Check sheet for the modelled part. Datum: model origin and axes. Units: mm. Give positions to 0.01 mm unless a question says otherwise; leave off trailing zeros. Loops run counter-clockwise (first coordinate to the right, second up) from the corner with the lowest first, then second, coordinate; pieces in that order, holes last. Notation, with made-up numbers: (-23, 82) - (29, 82) arc R14 cw to (29, 96) - close; hole circle Ø7 at (82.25, 19). An arc over 180 degrees is marked (long way). Answer in a Markdown table with one row per item. Add a question column.
(1) Go/stop test with a flat-tipped pin: P1, Ø1, axis at x = -98.5, z = 2, coming from the +Y side. Record where the tip stops, or that it passes through.
(2) Sectioned sample at C-C on z = 0.85. State how many separate pieces and enclosed holes the cut face has, then the cut area to 3 significant figures.
(3) Sectioned sample at B-B on x = -0.5. Enter the section's corners in (y, z).
(4) Thickness scan on L1, parallel to Y at x = -44.5, z = 0.6; L2, parallel to Y at x = 35, z = 1.3; L3, parallel to Y at x = -6.5, z = 2.15. Record the ranges inside material, lowest first.
(5) Sectioned sample at A-A on x = -146.5. Enter the section's corners in (y, z), then the cut area to 3 significant figures.
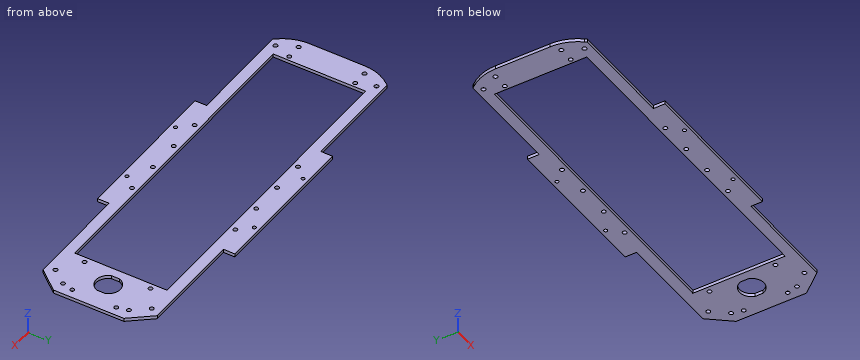
from build123d import *

# Parameters (mm, degrees)
BOSS_EXTRUDE1_DEPTH            = 3
SKETCH2_W                      = 285
SKETCH2_H                      = 84
CUT_EXTRUDE1_DEPTH             = 3
SKETCH3_R                      = 1.95
SKETCH3_R_2                    = 1.6
CUT_EXTRUDE2_DEPTH             = 3
CUT_EXTRUDE3_DEPTH             = 3
SKETCH5_R                      = 1.9
CUT_EXTRUDE4_DEPTH             = 3
SKETCH7_W                      = 36.585559037
SKETCH7_H                      = 111.194930045
CUT_EXTRUDE5_DEPTH             = 10
FILLET1_R                      = 40
SKETCH6_R                      = 1.9
EXPANSION_MOUNTING_HOLES_DEPTH = 10


with BuildPart() as part:
    # Sketch1 → Boss-Extrude1 (new body)
    with BuildSketch(Plane.XY):
        Polygon((-70, 89.297239119), (70, 89.297239119), (70, 78.797239119), (165, 78.797239119), (181.5, 58.797239119), (181.5, -5.202760881), (165, -25.202760881), (70, -25.202760881), (70, -35.702760881), (-70, -35.702760881), (-70, -25.202760881), (-165, -25.202760881), (-181.5, -5.202760881), (-181.5, 58.797239119), (-165, 78.797239119), (-70, 78.797239119), align=None)
    extrude(amount=BOSS_EXTRUDE1_DEPTH)

    # Sketch2 → Cut-Extrude1 (cut)
    with BuildSketch(Plane.XY.offset(3)):
        with Locations((-7.5, 26.797239119)):
            Rectangle(SKETCH2_W, SKETCH2_H)
    extrude(amount=-CUT_EXTRUDE1_DEPTH, mode=Mode.SUBTRACT)

    # Sketch3 → Cut-Extrude2 (cut)
    with BuildSketch(Plane.XY.offset(3)):
        with Locations((-167.5, -3.202760881)):
            Circle(SKETCH3_R)
        with Locations((-167.5, 56.797239119)):
            Circle(SKETCH3_R)
        with Locations((-35, -31.202760881)):
            Circle(SKETCH3_R_2)
        with Locations((35, -31.202760881)):
            Circle(SKETCH3_R_2)
        with Locations((-35, 84.797239119)):
            Circle(SKETCH3_R_2)
        with Locations((35, 84.797239119)):
            Circle(SKETCH3_R_2)
        with Locations((-159.5, 72.797239119)):
            Circle(SKETCH3_R)
        with Locations((-159.5, -19.202760881)):
            Circle(SKETCH3_R)
    extrude(amount=-CUT_EXTRUDE2_DEPTH, mode=Mode.SUBTRACT)

    # Sketch4 → Cut-Extrude3 (cut)
    with BuildSketch(Plane.XY.offset(3)):
        with BuildLine():
            Line((163.8, 30.531204839), (163.8, 23.063273399))
            ThreePointArc((163.8, 23.063273399), (153.4, 15.747239119), (143, 23.063273399))
            Line((143, 23.063273399), (143, 30.531204839))
            ThreePointArc((143, 30.531204839), (153.4, 37.847239119), (163.8, 30.531204839))
        make_face()
    extrude(amount=-CUT_EXTRUDE3_DEPTH, mode=Mode.SUBTRACT)

    # Sketch5 → Cut-Extrude4 (cut)
    with BuildSketch(Plane.XY.offset(3)):
        with Locations((173.5, 6.797239119)):
            Circle(SKETCH5_R)
        with Locations((173.5, 46.797239119)):
            Circle(SKETCH5_R)
        with Locations((140, 56.797239119)):
            Circle(SKETCH5_R)
        with Locations((140, -3.202760881)):
            Circle(SKETCH5_R)
        with Locations((160, 70.547239119)):
            Circle(SKETCH5_R)
        with Locations((160, -16.952760881)):
            Circle(SKETCH5_R)
    extrude(amount=-CUT_EXTRUDE4_DEPTH, mode=Mode.SUBTRACT)

    # Sketch7 → Cut-Extrude5 (cut)
    with BuildSketch(Plane.XY.offset(3)):
        with Locations((-193.792779519, 34.073054392)):
            Rectangle(SKETCH7_W, SKETCH7_H)
    extrude(amount=-CUT_EXTRUDE5_DEPTH, mode=Mode.SUBTRACT)

    # Fillet1
    fillet1_edges = [part.edges().sort_by_distance(p)[0] for p in [
        (-175.5, 66.069966392, 1.5),
        (-175.5, -12.475488154, 1.5),
    ]]
    fillet(fillet1_edges, radius=FILLET1_R)

    # Sketch6 → Expansion mounting holes (cut)
    with BuildSketch(Plane.XY.offset(3)):
        with Locations((171, 56.797239119)):
            Circle(SKETCH6_R)
        with Locations((171, -3.202760881)):
            Circle(SKETCH6_R)
        with Locations((-154, 56.797239119)):
            Circle(SKETCH6_R)
        with Locations((-154, -3.202760881)):
            Circle(SKETCH6_R)
        with Locations((-45, 73.797239119)):
            Circle(SKETCH6_R)
        with Locations((-45, -20.202760881)):
            Circle(SKETCH6_R)
        with Locations((-15, -20.202760881)):
            Circle(SKETCH6_R)
        with Locations((-15, 73.797239119)):
            Circle(SKETCH6_R)
        with Locations((15, -20.202760881)):
            Circle(SKETCH6_R)
        with Locations((15, 73.797239119)):
            Circle(SKETCH6_R)
        with Locations((45, -20.202760881)):
            Circle(SKETCH6_R)
        with Locations((45, 73.797239119)):
            Circle(SKETCH6_R)
    extrude(amount=-EXPANSION_MOUNTING_HOLES_DEPTH, mode=Mode.SUBTRACT)


solid = part.part
Reply:
| question | item | result |
|---|---|---|
| 1 | P1 | y = 78.8 |
| 2 | separate pieces | 1 |
| 2 | enclosed holes | 28 |
| 2 | area | 15,000 mm^2 |
| 3 | outline | (-35.7, 0) - (-15.2, 0) - (-15.2, 3) - (-35.7, 3) - close; (68.8, 0) - (89.3, 0) - (89.3, 3) - (68.8, 3) - close |
| 4 | L1 | -35.7 to -22.04, -18.37 to -15.2, 68.8 to 71.96, 75.63 to 89.3 |
| 4 | L2 | -35.7 to -32.8, -29.6 to -15.2, 68.8 to 83.2, 86.4 to 89.3 |
| 4 | L3 | -35.7 to -15.2, 68.8 to 89.3 |
| 5 | outline | (-25.2, 0) - (-15.2, 0) - (-15.2, 3) - (-25.2, 3) - close; (68.8, 0) - (78.8, 0) - (78.8, 3) - (68.8, 3) - close |
| 5 | area | 60.0 mm^2 |
